Autodesk Inventor part; units mm, degrees
ref_plane "YZ Plane" through (0, 0, 0) normal (1, 0, 0) x (0, 1, 0)
ref_plane "XZ Plane" through (0, 0, 0) normal (0, 1, 0) x (-1, 0, 0)
ref_plane "XY Plane" through (0, 0, 0) normal (0, 0, 1) x (1, 0, 0)
sketch "Sketch1" plane through (0, 0, 0) normal (0, 0, 1) x (1, 0, 0)
  point P0 (0, 0)
sketch "Sketch2" plane through (0, 0, 0) normal (0, 0, 1) x (1, 0, 0)
  point P0 (0, 0)
sketch "Sketch3" plane through (0, 0, 0) normal (0, 0, 1) x (1, 0, 0)
  line L0 (-51, -36) -> (51, -36)
  line L1 (51, -36) -> (51, 36)
  line L2 (51, 36) -> (-51, 36)
  line L3 (-51, 36) -> (-51, -36)
  line L4 (-51, -36) -> (51, 36) construction
  line L5 (51, -36) -> (-51, 36) construction
  line L6 (-55, 40) -> (55, 40)
  line L7 (55, 40) -> (55, -40)
  line L8 (55, -40) -> (-55, -40)
  line L9 (-55, -40) -> (-55, 40)
  line L10 (-55, 40) -> (55, -40) construction
  line L11 (55, 40) -> (-55, -40) construction
  point P0 (0, 0)
  dimension "d0" = 102
  dimension "d1" = 72
  dimension "d2" = 110
  dimension "d3" = 80
extrude "Extrusion1" add sketch "Sketch3" against normal blind 35
sketch "Sketch4" plane through (51, -36, 0) normal (-1, 0, 0) x (0, 0, 1)
  point P0 (0, 36)
sketch "Sketch5" plane through (-55, -40, 0) normal (-1, 0, 0) x (0, 0, 1)
  line L0 (0, 80) -> (-35, 80)
  line L1 (0, 0) -> (-35, 0)
  line L2 (-35, 80) -> (-30, 80)
  line L3 (-30, 80) -> (-30, 0)
  line L4 (-30, 0) -> (-35, 0)
  line L5 (-35, 0) -> (-35, 80)
  point P0 (0, 40)
  point P1 (-30, 80)
  dimension "d6" = 5
extrude "Extrusion2" add sketch "Sketch5" against normal blind 110
fillet "Fillet1" radius 2 8 edges at (-55, 40, -17.5) (0, 40, -35) (55, 40, -17.5) (-55, 0, -35) (-55, -40, -17.5) (0, -40, -35) (55, 0, -35) (55, -40, -17.5)
sketch "Sketch6" plane through (55, -38, 0) normal (1, 0, 0) x (0, 0, -1)
  line L0 (3, 2) -> (7, 2)
  line L1 (7, 2) -> (7, 74)
  line L2 (7, 74) -> (3, 74)
  line L3 (3, 74) -> (3, 2)
  line L4 (3, 2) -> (7, 74) construction
  line L5 (7, 2) -> (3, 74) construction
  line L6 (0, 0) -> (0, 76)
  line L7 (33, 0) -> (0, 0)
  point P0 (0, 38)
  point P1 (5, 38)
  point P2 (5, 74)
  dimension "d26" = 3
  dimension "d27" = 2
  dimension "d28" = 72
  dimension "d29" = 4
extrude "Extrusion3" cut sketch "Sketch6" against normal blind 10
sketch "Sketch7" plane through (-51, 36, 0) normal (0, -1, 0) x (1, 0, 0)
  point P0 (51, 0)
sketch "Sketch11" plane through (-51, 36, -30) normal (0, 0, 1) x (1, 0, 0)
  circle A0 centre (2.54, -2.54) radius 1.27
  line L0 (0, 0) -> (102, 0)
  line L1 (0, -72) -> (0, 0)
  circle A1 centre (2.54, -21.59) radius 1.27
  point P0 (51, -36)
  dimension "d44" = 2.54
  dimension "d45" = 2.54
  dimension "d46" = 2.54
  dimension "d47" = 2.54
  dimension "d48" = 2.54
  dimension "d49" = 19.05
extrude "Extrusion6" add sketch "Sketch11" along normal blind 2
sketch "Sketch12" plane through (-55, -38, 0) normal (-1, 0, 0) x (0, 0, 1)
  point P0 (0, 38)
sketch "Sketch13" plane through (-55, -38, 0) normal (-1, 0, 0) x (0, 0, 1)
  line L0 (0, 76) -> (0, 0)
  line L1 (0, 76) -> (-8, 76)
  line L2 (-8, 76) -> (-8, 0)
  line L3 (-8, 0) -> (0, 0)
  line L4 (0, 0) -> (0, 76)
  point P0 (0, 38)
  point P1 (-4, 0)
  point P2 (-4, 76)
  dimension "d52" = 8
  dimension "d53" = 76
extrude "Extrusion7" add sketch "Sketch13" against normal blind 110
sketch "Sketch14" plane through (55, -38, 0) normal (1, 0, 0) x (0, 0, -1)
  line L0 (2, 2) -> (5, 2)
  line L1 (5, 2) -> (5, 74)
  line L2 (5, 74) -> (2, 74)
  line L3 (2, 74) -> (2, 2)
  line L4 (0, 0) -> (0, 76)
  line L5 (33, 0) -> (0, 0)
  point P0 (0, 38)
  point P1 (3.5, 2)
  dimension "d56" = 3
  dimension "d57" = 2
  dimension "d58" = 72
  dimension "d59" = 2
extrude "Extrusion8" cut sketch "Sketch14" against normal blind 106
sketch "Sketch15" plane through (0, 0, 0) normal (0, 0, 1) x (1, 0, 0)
  line L0 (-51, 34) -> (51, 34)
  line L1 (51, 34) -> (51, -34)
  line L2 (51, -34) -> (-51, -34)
  line L3 (-51, -34) -> (-51, 34)
  line L4 (-51, 34) -> (51, -34) construction
  line L5 (51, 34) -> (-51, -34) construction
  point P0 (0, 0)
  dimension "d62" = 102
  dimension "d63" = 68
extrude "Extrusion9" cut sketch "Sketch15" against normal blind 10
sketch "Sketch16" plane through (-51, -36, -30) normal (1, 0, 0) x (0, 0, -1)
  point P0 (-30, 36)
sketch "Sketch17" plane through (-55, -38, 0) normal (-1, 0, 0) x (0, 0, 1)
  line L0 (-11, 27) -> (-15, 27)
  line L1 (-15, 27) -> (-15, 2)
  line L2 (-15, 2) -> (-11, 2)
  line L3 (-11, 2) -> (-11, 27)
  line L4 (0, 76) -> (0, 0)
  line L5 (0, 0) -> (-33, 0)
  point P0 (0, 38)
  point P1 (-13, 2)
  point P2 (-13, 27)
  dimension "d96" = 11
  dimension "d97" = 2
  dimension "d98" = 4
  dimension "d99" = 25
extrude "Extrusion10" add sketch "Sketch17" against normal blind 16
sketch "Sketch18" plane through (-51, -36, -11) normal (0, 0, 1) x (1, 0, 0)
  point P0 (51, 36)
sketch "Sketch19" plane through (-51, 36, -30) normal (0, 0, 1) x (1, 0, 0)
  circle A0 centre (74.07, -11.97) radius 1.5
  line L0 (102, 0) -> (102, -72)
  line L1 (0, 0) -> (102, 0)
  circle A1 centre (72.8, -60.03) radius 1.5
  line L2 (102, -72) -> (0, -72)
  circle A2 centre (74.07, -11.97) radius 3.5
  circle A3 centre (72.8, -60.03) radius 3.5
  point P0 (51, -36)
  dimension "d102" = 3
  dimension "d103" = 27.93
  dimension "d104" = 11.97
  dimension "d105" = 3
  dimension "d106" = 29.2
  dimension "d107" = 11.97
  dimension "d108" = 7
  dimension "d109" = 7
extrude "Extrusion11" add sketch "Sketch19" along normal blind 9.03
sketch "Sketch20" plane through (-53, 40, 0) normal (0, 1, 0) x (1, 0, 0)
  point P0 (53, 0)
sketch "Sketch21" plane through (-53, 40, 0) normal (0, 1, 0) x (1, 0, 0)
  circle A0 centre (16, 14) radius 1.95
  line L0 (106, 0) -> (0, 0)
  line L1 (106, 33) -> (106, 0)
  circle A1 centre (8, 14) radius 1.95
  point P0 (53, 0)
  dimension "d116" = 3.9
  dimension "d117" = 14
  dimension "d118" = 90
  dimension "d119" = 3.9
  dimension "d120" = 8
  dimension "d121" = 14
extrude "Extrusion12" cut sketch "Sketch21" against normal blind 10
sketch "Sketch22" plane through (55, -38, 0) normal (1, 0, 0) x (0, 0, -1)
  line L0 (16.43, 21.99) -> (20.33, 21.99)
  line L1 (20.33, 21.99) -> (20.33, 29.69)
  line L2 (20.33, 29.69) -> (16.43, 29.69)
  line L3 (16.43, 29.69) -> (16.43, 21.99)
  line L4 (33, 0) -> (0, 0)
  line L5 (5, 74) -> (5, 2)
  point P0 (0, 38)
  point P1 (18.38, 21.99)
  point P2 (16.43, 25.84)
  dimension "d140" = 21.99
  dimension "d141" = 3.9
  dimension "d142" = 7.7
  dimension "d143" = 11.43
extrude "Extrusion13" cut sketch "Sketch22" against normal blind 10
sketch "Sketch8" plane through (-53, -40, 0) normal (0, -1, 0) x (1, 0, 0)
  line L0 (2, 0) -> (104, 0)
  line L1 (104, 0) -> (104, -3)
  line L2 (104, -3) -> (2, -3)
  line L3 (2, -3) -> (2, 0)
  line L4 (0, 0) -> (106, 0)
  line L5 (0, -33) -> (0, 0)
  point P0 (53, 0)
  point P1 (2, -1.5)
  point P2 (104, -1.5)
  dimension "d32" = 0
  dimension "d33" = 3
  dimension "d34" = 2
  dimension "d35" = 102
sketch "Sketch9" plane through (0, 0, 0) normal (0, 0, 1) x (1, 0, 0)
  line L0 (-51, 35) -> (51, 35)
  line L1 (51, 35) -> (51, -35)
  line L2 (51, -35) -> (-51, -35)
  line L3 (-51, -35) -> (-51, 35)
  line L4 (-51, 35) -> (51, -35) construction
  line L5 (51, 35) -> (-51, -35) construction
  point P0 (0, 0)
  dimension "d39" = 102
  dimension "d40" = 70
properties part number "BoxV2"
Could you check a few things on this model? Use its own coordinates, in mm. A direction names the side the tool comes from. Round coordinates to 2 decimals unless told otherwise and drop trailing zeros. Order: outer loops, then holes, each group sorted by start corner. A loop starts at its lowest first (then second) coordinate and runs counter-clockwise, first axis right, second up. Notation, with made-up numbers: M 28,32 L 59,32 A29 cw 59,54 Z; hole C 89,12 d5. An arc over 180 degrees is marked long. One line per item, written item: value.
(1) If we mould it in two halves opening along X, with no side actions, what happens to faces 4 (the cylindrical face through (22.311, 27.447, -25.548)), 5 (the cylindrical face through (-49.47, 34.23, -29.01)), 6 (the flat face through (3, 36, -4))? For each: released by +X, released by -X, zero draft, split by the parting line, or undercut.
Ans:
face 4: undercut
face 5: undercut
face 6: zero draft
(2) I need wall thicknesses on line 1 along Y through (x, z) = (-13, -13); line 2 along X through (y, z) = (21, -6); line 3 along Y through (x, z) = (21.8, -23.5). Which ranges of each line are inside material? Lowest first, please. Write a range as from..to.
Ans:
line 1: y = -40..-36, 36..40
line 2: x = -55..-51, 51..55
line 3: y = -40..-36, -27.53..-25.53, -22.53..-20.53, 20.77..23.23, 24.83..27.29, 36..40
(3) I'm going to push flat-ended pins straight in: P1, Ø0.9, axis at x = 22.5, y = -23.5, coming from the +Z side; P2, Ø5, axis at x = 23.07, y = 24.03, coming from the +Z side. Where does each tip first touch, or does it pass through?
Ans:
P1: stops at z = -30
P2: stops at z = -20.97
(4) Imagine slicing it at C-C (z = -18). Write out the boundary of the cut face in (x, y).
Ans:
outline: M -55,-38 A2 ccw -53,-40 L 53,-40 A2 ccw 55,-38 L 55,-16.01 L 51,-16.01 L 51,-36 L -51,-36 L -51,36 L 51,36 L 51,-8.31 L 55,-8.31 L 55,38 A2 ccw 53,40 L -53,40 A2 ccw -55,38 Z
(5) Imagine slicing it at D-D (x = 43). Write out the boundary of the cut face in (y, z), and give its area (3 significant figures).
Ans:
outline: M -40,-33 A2 ccw -38,-35 L 38,-35 A2 ccw 40,-33 L 40,0 L 34,0 L 34,-2 L 36,-2 L 36,-5 L 34,-5 L 34,-8 L 36,-8 L 36,-30 L -36,-30 L -36,-8 L -34,-8 L -34,-5 L -36,-5 L -36,-2 L -34,-2 L -34,0 L -40,0 Z
area: 658 mm^2
(6) Imagine slicing it at B-B (y = -1). Write out the boundary of the cut face in (x, z).
Ans:
outline: M -55,-33 A2 ccw -53,-35 L 53,-35 A2 ccw 55,-33 L 55,-5 L 51,-5 L 51,-30 L -51,-30 L -51,0 L -55,0 Z; M 51,-2 L 55,-2 L 55,0 L 51,0 Z
(7) Which directions (+Z, -Z, +X, -X, +Y, -Y) give clear straight access to the entire face, cutting with the end or side of a thin tool? Please do faces 1 (the flat face through (53, -12, -16.43)), 2 (the flat face through (-48, 14, -28)), 3 (the cylindrical face through (-43.2, 38.03, -13.25)).
Ans:
face 1: +X
face 2: +Z
face 3: +Y
